```python
from build123d import *

# Parameters (mm, degrees)
F1_DEPTH = 20
F2_R     = 5
F3_R     = 5
F4_ANGLE = 90


with BuildPart() as f1:
    # F0 (on Front) → F1 (new body)
    with BuildSketch(Plane.XZ):
        with BuildLine():
            Line((32, 38.04), (5, 38.04))
            ThreePointArc((5, 38.04), (1.4644660941, 36.5755339059), (0, 33.04))
            Line((0, 33.04), (0, 28.04))
            Line((0, 28.04), (20, 28.04))
            ThreePointArc((20, 28.04), (23.5355339059, 26.5755339059), (25, 23.04))
            Line((25, 23.04), (25, 15))
            ThreePointArc((25, 15), (23.5355339059, 11.4644660941), (20, 10))
            Line((20, 10), (0, 10))
            Line((0, 10), (0, 0))
            Line((0, 0), (72, 0))
            ThreePointArc((72, 0), (75.5355339059, 1.4644660941), (77, 5))
            Line((77, 5), (77, 20))
            Line((77, 20), (67, 20))
            Line((67, 20), (67, 17))
            ThreePointArc((67, 17), (65.5355339059, 13.4644660941), (62, 12))
            Line((62, 12), (42, 12))
            ThreePointArc((42, 12), (38.4644660941, 13.4644660941), (37, 17))
            Line((37, 17), (37, 33.04))
            ThreePointArc((37, 33.04), (35.5355339059, 36.5755339059), (32, 38.04))
        make_face()
    extrude(amount=F1_DEPTH)

    # F2
    f2_edges = [f1.edges().sort_by_distance(p)[0] for p in [
        (67, -10, 20),
    ]]
    fillet(f2_edges, radius=F2_R)

    # F3
    f3_edges = [f1.edges().sort_by_distance(p)[0] for p in [
        (77, -10, 20),
    ]]
    fillet(f3_edges, radius=F3_R)


with BuildPart() as f1_1:
    # F4: moved
    add(f1.part.rotate(Axis((36, 0, 0), (-1, 0, 0)), F4_ANGLE))


solid = f1_1.part
```
Geometry: final body of the model. Coordinates: model frame, mm. A direction names the side the tool comes from. Coordinates: 2 decimals unless noted, no trailing zeros. Order: outer loops, then holes, each group sorted by start corner. A loop starts at its lowest first (then second) coordinate and runs counter-clockwise, first axis right, second up. Notation, with made-up numbers: (37, -16) - (75, -16) arc R25 cw to (75, 10) - close; hole circle Ø8 at (52.5, 14.5). An arc over 180 degrees is marked (long way). Write each question's results on one line, items separated by ' | '.
1) Section A-A, the plane x = 7.5. Return loops of the section in (y, z).
Results list:
outline: (0, 0) - (10, 0) - (10, 20) - (0, 20) - close; (28.04, 0) - (38.04, 0) - (38.04, 20) - (28.04, 20) - close
2) Section C-C, the plane y = 29. Return loops of the section in (x, z), plus the area to 3 significant figures.
Results list:
outline: (0, 0) - (37, 0) - (37, 20) - (0, 20) - close | area: 740 mm^2
3) Section D-D, the plane x = 51.5. Return loops of the section in (y, z).
Results list:
outline: (0, 0) - (12, 0) - (12, 20) - (0, 20) - close
4) Pull-direction query (Y, two-part tool) for faces 1 (the cylindrical face through (39, 13, 10)), 2 (the flat face through (77, 10, 10)), 3 (the cylindrical face through (24, 12, 10)); classes: pulls with the +Y half, pulls with the -Y half, needs draft (parallel to the pull), parting line crosses it, or undercut.
Results list:
face 1: pulls with the +Y half | face 2: needs draft | face 3: undercut
5) Section B-B, the plane y = 14. Return loops of the section in (x, z).
Results list:
outline: (24.9, 0) - (38, 0) - (38, 20) - (24.9, 20) - close; (66, 0) - (77, 0) - (77, 20) - (66, 20) - close
6) Pin query (flat end, axial travel): pin 1 (4 mm diameter, centred on y = 20, z = 5.5, fed in from -X); pin 2 (12 mm diameter, centred on x = 59.5, z = 14.5, fed in from +Y); pin 3 (10 mm diameter, centred on y = 29.5, z = 6, fed in from +X). Return the tip coordinate at first contact, or that it passes through.
Results list:
pin 1: x = 25 | pin 2: y = 13.43 | pin 3: x = 37
7) Line query: line 1 (Y direction, x = 13, z = 7.75); line 2 (X direction, y = 30, z = 18.5); line 3 (Y direction, x = 60, z = 18.75). Output: solid intervals per line, ascending. Write a range as from..to.
Results list:
line 1: 0..10, 28.04..38.04 | line 2: 0..37 | line 3: 0..12
8) Set-up query: faces 4 (the flat face through (19, 38.04, 10)), 5 (the flat face through (37, 25, 10)), 6 (the flat face through (10, 10, 10)). Return all of +Z, -Z, +X, -X, +Y, -Y with unobstructed straight access to the full face (end or side cutting, diameter ignored); none if empty.
Results list:
face 4: +Z, -Z, +X, -X, +Y | face 5: +Z, -Z, +Y | face 6: +Z, -Z, -X
